Build history of the part. All positions in model axes, mm. Coordinates: 2 decimals unless noted, no trailing zeros. Order: outer loops, then holes, each group sorted by start corner. A loop starts at its lowest first (then second) coordinate and runs counter-clockwise, first axis right, second up. Notation, with made-up numbers: (83.25, 68.5) - (122.25, 68.5) arc R28 ccw to (122.25, 89.5) - close; hole circle Ø11 at (77.5, 83). An arc over 180 degrees is marked (long way). Return JSON: item names as keys, results as strings.
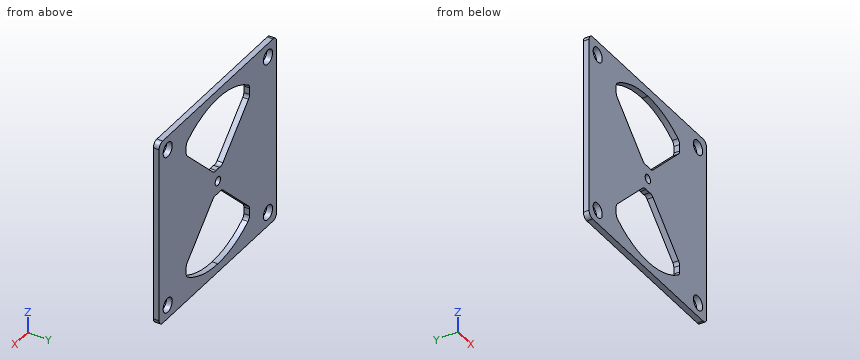
Autodesk Inventor part; units mm, degrees
ref_plane "YZ Plane" through (0, 0, 0) normal (1, 0, 0) x (0, 1, 0)
ref_plane "XZ Plane" through (0, 0, 0) normal (0, 1, 0) x (-1, 0, 0)
ref_plane "XY Plane" through (0, 0, 0) normal (0, 0, 1) x (1, 0, 0)
sketch "Sketch1" plane through (0, 0, 0) normal (0, 1, 0) x (-1, 0, 0)
  arc A0 (20.126, -22.2473) -> (-20.126, -22.2473) centre (0, 0) ccw construction
  circle A1 centre (0, 0) radius 33 construction
  line L0 (33, 33) -> (-33, 33)
  line L1 (-33, 33) -> (-33, -33)
  line L2 (-33, -33) -> (33, -33)
  line L3 (33, -33) -> (33, 33)
  line L4 (33, 33) -> (23.3345, 23.3345) construction
  line L5 (-33, 33) -> (-23.3345, 23.3345) construction
  line L6 (23.3345, 23.3345) -> (-23.3345, -23.3345) construction
  line L7 (23.3345, -23.3345) -> (33, -33) construction
  line L8 (-23.3345, -23.3345) -> (-33, -33) construction
  line L9 (-23.3345, 23.3345) -> (23.3345, -23.3345) construction
  line L10 (0, -33) -> (0, 33) construction
  line L11 (33, 0) -> (-33, 0) construction
  circle A2 centre (0, 0) radius 1.5
  circle A3 centre (0, 0) radius 4.5
  line L12 (4.0607, -1.9393) -> (22.2473, -20.126) construction
  line L13 (1.9393, -4.0607) -> (17.8, -19.9213)
  arc A4 (0, -30) -> (17.8, -24.1487) centre (0, 0) ccw
  line L14 (23.3345, 23.3345) -> (-23.3345, -23.3345) construction
  line L15 (-4.0607, -1.9393) -> (-22.2473, -20.126) construction
  line L16 (-1.9393, -4.0607) -> (-17.8, -19.9213)
  arc A5 (-20.126, -22.2473) -> (-17.8, -24.1487) centre (0, 0) ccw construction
  line L17 (17.8, -24.1487) -> (17.8, -19.9213)
  line L18 (-17.8, -24.1487) -> (-17.8, -19.9213)
  line L19 (17.8, -22.035) -> (-17.8, -22.035) construction
  arc A6 (-17.8, -24.1487) -> (0, -30) centre (0, 0) ccw
  line L20 (-17.8, -19.9213) -> (-20.126, -22.2473) construction
  line L21 (17.8, -19.9213) -> (20.126, -22.2473) construction
  arc A7 (17.8, -24.1487) -> (20.126, -22.2473) centre (0, 0) ccw construction
  line L22 (1.9393, 4.0607) -> (17.8, 19.9213)
  arc A8 (17.8, 24.1487) -> (0, 30) centre (0, 0) ccw
  line L23 (-1.9393, 4.0607) -> (-17.8, 19.9213)
  arc A9 (-17.8, 24.1487) -> (-20.126, 22.2473) centre (0, 0) ccw construction
  line L24 (17.8, 24.1487) -> (17.8, 19.9213)
  line L25 (-17.8, 24.1487) -> (-17.8, 19.9213)
  arc A10 (0, 30) -> (-17.8, 24.1487) centre (0, 0) ccw
  line L26 (-17.8, 19.9213) -> (-20.126, 22.2473) construction
  line L27 (17.8, 19.9213) -> (20.126, 22.2473) construction
  arc A11 (20.126, 22.2473) -> (17.8, 24.1487) centre (0, 0) ccw construction
  circle A12 centre (28.1673, -28.1673) radius 2.55
  circle A13 centre (-28.1673, -28.1673) radius 2.55
  circle A14 centre (-28.1673, 28.1673) radius 2.55
  circle A15 centre (28.1673, 28.1673) radius 2.55
  point P0 (0, -22.035)
  dimension "d22" = 60
  dimension "d24" = 3
  dimension "d25" = 3
  dimension "d26" = 3
  dimension "d27" = 1.5
  dimension "d28" = 3
  dimension "d31" = 35.6
  dimension "d32" = 5.1
  dimension "d33" = 5.1
  dimension "d34" = 5.1
  dimension "d35" = 5.1
extrude "Extrusion1" add sketch "Sketch1" along normal blind 2 contours L3 L2 L1 L0 | A3
fillet "Fillet3" radius 2 16 edges at (-17.8, 1, 19.9213) (-1.9393, 1, 4.0607) (1.9393, 1, 4.0607) (-17.8, 1, 24.1487) (17.8, 1, 24.1487) (17.8, 1, 19.9213) (-1.9393, 1, -4.0607) (1.9393, 1, -4.0607) (17.8, 1, -19.9213) (17.8, 1, -24.1487) (-17.8, 1, -19.9213) (-17.8, 1, -24.1487) (-33, 1, 33) (-33, 1, -33) (33, 1, -33) (33, 1, 33)
properties part number "Feeder Bottom Plate" material "Aluminum 6061"
1. Drop flat-ended pins along their axis: pin 1 (2.5 mm diameter, centred on x = 0, z = 0, fed in from -Y); pin 2 (2 mm diameter, centred on x = -13, z = -14, fed in from -Y). Give the stop position or say it passes through.
Check values:
{"pin 1": "through", "pin 2": "y = 0"}
2. Cut at A-A on z = 0. Give the cut face in (x, y), plus the area to 3 significant figures.
Check values:
{"outline": "(-33, 0) - (-1.5, 0) - (-1.5, 2) - (-33, 2) - close; (1.5, 0) - (33, 0) - (33, 2) - (1.5, 2) - close", "area": "126 mm²"}
3. Cut at B-B on x = -27. Give the cut face in (y, z).
Check values:
{"outline": "(0, -33) - (2, -33) - (2, -30.43) - (0, -30.43) - close; (0, -25.9) - (2, -25.9) - (2, 25.9) - (0, 25.9) - close; (0, 30.43) - (2, 30.43) - (2, 33) - (0, 33) - close"}
4. Cut at C-C on y = 1. State how many separate pieces and enclosed holes the cut face has, plus the area to 3 significant figures.
Check values:
{"separate pieces": "1", "enclosed holes": "7", "area": "3,060 mm²"}
5. Probe L1, parallel to Z at x = 28, y = 1.35; L2, parallel to X at y = 0.7, z = 22.5; L3, parallel to Z at x = 14.5, y = 1.05. List the from-to ranges inside material, lowest first.
Check values:
{"L1": "-33 to -30.71, -25.62 to 25.62, 30.71 to 33", "L2": "-33 to -17.8, 17.8 to 33", "L3": "-33 to -26.26, -16.62 to 16.62, 26.26 to 33"}
6. Cut at D-D on x = 6. Give the cut face in (y, z), plus the area to 3 significant figures.
Check values:
{"outline": "(0, -33) - (2, -33) - (2, -29.39) - (0, -29.39) - close; (0, -8.12) - (2, -8.12) - (2, 8.12) - (0, 8.12) - close; (0, 29.39) - (2, 29.39) - (2, 33) - (0, 33) - close", "area": "46.9 mm²"}
